from build123d import *

# Parameters (mm, degrees)
SKETCH2_W                    = 50.8
SKETCH2_H                    = 25.4
BOSS_EXTRUDE1_DEPTH          = 3.175
CUT_EXTRUDE2_DEPTH           = 4.175
FILLET2_R                    = 3.175
SKETCH5_W                    = 3.429
SKETCH5_H                    = 9.779
SKETCH5_H_2                  = 12.954
CUT_EXTRUDE3_DEPTH           = 4.175
F_10_0_1935_DIAMETER_HOLE1_D = 4.9149


with BuildPart() as part:
    # Sketch2 → Boss-Extrude1 (new body)
    with BuildSketch(Plane(origin=(0, 0, 0), x_dir=(0, 0, -1), z_dir=(1, 0, 0))):
        Rectangle(SKETCH2_W, SKETCH2_H)
    extrude(amount=BOSS_EXTRUDE1_DEPTH)

    # Sketch4 → Cut-Extrude2 (cut, through all)
    with BuildSketch(Plane(origin=(3.175, 0, 0), x_dir=(0, 0, -1), z_dir=(1, 0, 0))):
        Polygon((0, -12.98702), (-25.4, -12.7), (-46.852380557, -12.7), (-46.852380557, 5.701326041), (-22.403810306, -4.050651033), align=None)
    extrude(amount=-CUT_EXTRUDE2_DEPTH, mode=Mode.SUBTRACT)

    # Fillet2
    fillet2_edges = [part.edges().sort_by_distance(p)[0] for p in [
        (1.5875, -2.855539298, 25.4),
        (1.5875, 12.7, 25.4),
        (1.5875, 12.7, -25.4),
        (1.5875, -12.7, -25.4),
    ]]
    fillet(fillet2_edges, radius=FILLET2_R)

    # Sketch5 → Cut-Extrude3 (cut, through all)
    with BuildSketch(Plane(origin=(3.175, 0, 0), x_dir=(0, 0, -1), z_dir=(1, 0, 0))):
        with Locations((-12.8651, 3.048)):
            Rectangle(SKETCH5_W, SKETCH5_H)
        with Locations((12.8651, 0)):
            Rectangle(SKETCH5_W, SKETCH5_H_2)
    extrude(amount=-CUT_EXTRUDE3_DEPTH, mode=Mode.SUBTRACT)

    # #10 (0.1935) Diameter Hole1 (through all)
    with Locations(Plane(origin=(3.175, 0, 0), x_dir=(0, 0, -1), z_dir=(1, 0, 0))):
        with Locations((-19.05, 3.81), (0, -6.35), (0, 6.35)):
            Hole(F_10_0_1935_DIAMETER_HOLE1_D / 2)


solid = part.part
For this review, take the finished solid that the model builds, in its own axes (mm). A direction names the side the tool comes from. Give positions to 0.01 mm unless a question says otherwise; leave off trailing zeros. Loops run counter-clockwise (first coordinate to the right, second up) from the corner with the lowest first, then second, coordinate; pieces in that order, holes last.
Item 1: For line 1 along Y through (x, z) = (1.1, 0); line 2 along Z through (x, y) = (2.4, 1); line 3 along Y through (x, z) = (1.4, -11.5), list the stretches that pass through material, from the lowest coordinate up.
Item 2: Take a section at C-C, the plane y = -5.5. State the section outline as (x, z) points (3 decimals), and give its area (3 significant figures).
Item 3: Take a section at B-B, the plane x = 1.6. Give the number of separate pieces and of enclosed holes in the cut face, and give its area (3 significant figures).
Item 4: Take a section at A-A, the plane z = 0. State the section outline as (x, y) points (3 decimals).
Item 5: Insertion check: pin 1 (1.5 mm diameter, centred on x = 1, z = 4.5, fed in from -Y). The pin has a flat end and moves straight along its axis. Give the tip position at first contact, or say it passes through.
Item 6: Take a section at D-D, the plane z = 19.05. State the section outline as (x, y) points (3 decimals).
Item 7: Draft analysis for pull direction Y (two halves, no side actions). For faces 3 (the flat face through (3.175, 0, 0)), 4 (the flat face through (2, -1.842, 13)), 5 (the cylindrical face through (1.61, 11.75, 24.49)), 6 (the cylindrical face through (1.565, -3.913, -0.32)), state which applies: +Y half, -Y half, draft (parallel to the pull), parting line (faces both ways), or undercut.
Item 8: Tool access review of faces 1 (the flat face through (2, -12.7, -11)), 2 (the flat face through (2, 3, 11.151)): name each direction out of +Z, -Z, +X, -X, +Y, -Y from which nothing blocks a thin tool from reaching the whole face with its end or side.
Calculated:
1. line 1: y = -12.7 to -8.81, -3.89 to 3.89, 8.81 to 12.7
1. line 2: z = -25.4 to -14.58, -11.15 to 11.15, 14.58 to 25.4
1. line 3: y = -12.7 to -6.48, 6.48 to 12.7
2. outline: (0, -25.4) - (3.175, -25.4) - (3.175, -14.58) - (0, -14.58) - close; (0, -11.151) - (3.175, -11.151) - (3.175, -2.306) - (0, -2.306) - close; (0, 2.306) - (3.175, 2.306) - (3.175, 18.77) - (0, 18.77) - close
2. area: 115 mm2
3. separate pieces: 1
3. enclosed holes: 5
3. area: 1,030 mm2
4. outline: (0, -12.7) - (3.175, -12.7) - (3.175, -8.807) - (0, -8.807) - close; (0, -3.893) - (3.175, -3.893) - (3.175, 3.893) - (0, 3.893) - close; (0, 8.807) - (3.175, 8.807) - (3.175, 12.7) - (0, 12.7) - close
5. pin 1: stops at y = -11.49
6. outline: (0, -5.388) - (3.175, -5.388) - (3.175, 1.353) - (0, 1.353) - close; (0, 6.267) - (3.175, 6.267) - (3.175, 12.7) - (0, 12.7) - close
7. face 3: draft
7. face 4: undercut
7. face 5: +Y half
7. face 6: undercut
8. face 1: +Z, -Z, +X, -X, -Y
8. face 2: +X, -X
